from build123d import *
from OCP.BRepFilletAPI import BRepFilletAPI_MakeChamfer

# Parameters (mm, degrees)
SKETCH_1_W          = 46
SKETCH_1_H          = 21.3
EXTRUDE_1_DEPTH     = 2
SKETCH_2_R          = 8.3
CUT_EXTRUDE_1_DEPTH = 26.424840216
SKETCH_3_W          = 8
SKETCH_3_H          = 3
CUT_EXTRUDE_2_DEPTH = 26.424840216
SKETCH_4_W          = 5
SKETCH_4_H          = 4
CUT_EXTRUDE_3_DEPTH = 26.424840216
SKETCH_5_W          = 3
SKETCH_5_H          = 2
SKETCH_5_W_2        = 2
SKETCH_5_H_2        = 3
CUT_EXTRUDE_4_DEPTH = 1
SKETCH_8_W          = 46
SKETCH_8_H          = 2
EXTRUDE_2_DEPTH     = 5
SKETCH_9_W          = 46
SKETCH_9_H          = 14
EXTRUDE_3_DEPTH     = 3
HOLE_WIZARD_M3_1_D  = 3.4
HOLE_WIZARD_M4_1_D  = 4.5
RIB_1_REACH         = 34.754
SKETCH_13_WALL_W    = 79.877255328
SKETCH_13_WALL_H    = 8
CHAMFER_1_SIZE      = 8
CHAMFER_1_SIZE2     = 4.618802154


with BuildPart() as part:
    # 草圖1 → 填料-伸長1 (new body)
    with BuildSketch(Plane.XY):
        Rectangle(SKETCH_1_W, SKETCH_1_H)
    extrude(amount=EXTRUDE_1_DEPTH)

    # 草圖2 → 除料-伸長1 (cut, through all)
    with BuildSketch(Plane.XY.offset(2)):
        with Locations((-12.7, 0)):
            Circle(SKETCH_2_R)
        with Locations((12.7, 0)):
            Circle(SKETCH_2_R)
    extrude(amount=-CUT_EXTRUDE_1_DEPTH, mode=Mode.SUBTRACT)

    # 草圖3 → 除料-伸長2 (cut, through all)
    with BuildSketch(Plane.XY.offset(2)):
        with Locations((0, 9.15)):
            Rectangle(SKETCH_3_W, SKETCH_3_H)
    extrude(amount=-CUT_EXTRUDE_2_DEPTH, mode=Mode.SUBTRACT)

    # 草圖4 → 除料-伸長3 (cut, through all)
    with BuildSketch(Plane.XY.offset(2)):
        with Locations((0, -5.5)):
            Rectangle(SKETCH_4_W, SKETCH_4_H)
    extrude(amount=-CUT_EXTRUDE_3_DEPTH, mode=Mode.SUBTRACT)

    # 草圖5 → 除料-伸長4 (cut)
    with BuildSketch(Plane.XY.offset(2)):
        with Locations((4, -6.5)):
            Rectangle(SKETCH_5_W, SKETCH_5_H)
        with Locations((-5.5, 8.65)):
            Rectangle(SKETCH_5_W_2, SKETCH_5_H_2)
        with Locations((5.5, 8.65)):
            Rectangle(SKETCH_5_W_2, SKETCH_5_H_2)
    extrude(amount=-CUT_EXTRUDE_4_DEPTH, mode=Mode.SUBTRACT)

    # 草圖8 → 填料-伸長2 (add)
    with BuildSketch(Plane.XZ.offset(10.65)):
        with Locations((0, 1)):
            Rectangle(SKETCH_8_W, SKETCH_8_H)
    extrude(amount=EXTRUDE_2_DEPTH)

    # 草圖9 → 填料-伸長3 (add)
    with BuildSketch(Plane.XZ.offset(15.65)):
        with Locations((0, 7)):
            Rectangle(SKETCH_9_W, SKETCH_9_H)
    extrude(amount=EXTRUDE_3_DEPTH)

    # M3 餘隙孔1 (through all)
    with Locations(Plane.XY.offset(2)):
        with Locations((20.7, 8.6), (-20.7, -8.6), (-20.7, 8.6), (20.7, -8.6)):
            Hole(HOLE_WIZARD_M3_1_D / 2)

    # M4 餘隙孔1 (through all)
    with Locations(Plane(origin=(0, -15.65, 0), x_dir=(1, 0, 0), z_dir=(0, 1, 0))):
        with Locations((12, -10), (-12, -10)):
            Hole(HOLE_WIZARD_M4_1_D / 2)

    # 草圖13 wall → 肋材1 (add, up to next)
    with BuildSketch(Plane(origin=(0, -14.15, 8), x_dir=(0, -0.242535625036, 0.970142500145), z_dir=(0, -0.970142500145, -0.242535625036)), mode=Mode.PRIVATE) as rib_1_sk1:
        Rectangle(SKETCH_13_WALL_W, SKETCH_13_WALL_H)
    rib_1_tool1 = extrude(rib_1_sk1.sketch, amount=RIB_1_REACH, mode=Mode.PRIVATE) - part.part
    add(rib_1_tool1.solids().sort_by_distance((0, -14.15, 8))[0])

    # 導角1: one chamfer whose edges measure the first distance from different faces: ONE call of the kernel's chamfer builder (chamfer() names one face for all edges)
    chamfer_1_edges_1 = [part.edges().sort_by_distance(p)[0] for p in [
        (-23, -17.15, 14),
    ]]
    chamfer_1_side_1 = [part.faces().sort_by_distance(p)[0] for p in [
        (-23, 10.325270882, 1),
    ]]
    chamfer_1_edges_2 = [part.edges().sort_by_distance(p)[0] for p in [
        (23, -17.15, 14),
    ]]
    chamfer_1_side_2 = [part.faces().sort_by_distance(p)[0] for p in [
        (23, 10.325270882, 1),
    ]]
    chamfer_1 = BRepFilletAPI_MakeChamfer(part.part.solid().wrapped)
    for e in chamfer_1_edges_1:
        chamfer_1.Add(CHAMFER_1_SIZE, CHAMFER_1_SIZE2, e.wrapped, chamfer_1_side_1[0].wrapped)  # the first distance lies on this face
    for e in chamfer_1_edges_2:
        chamfer_1.Add(CHAMFER_1_SIZE, CHAMFER_1_SIZE2, e.wrapped, chamfer_1_side_2[0].wrapped)  # the first distance lies on this face
    add(Compound.cast(chamfer_1.Shape()), mode=Mode.REPLACE)


solid = part.part
Verification items for the finished model (mm, model axes). A direction names the side the tool comes from. Round coordinates to 2 decimals unless told otherwise and drop trailing zeros. Loops run counter-clockwise (first coordinate to the right, second up) from the corner with the lowest first, then second, coordinate; pieces in that order, holes last. Notation, with made-up numbers: M -26.5,62 L 10.5,62 A17 cw 10.5,81 Z; hole C 55.25,4 d4. An arc over 180 degrees is marked long. Write each question's results on one line, items separated by ' | '.
1) Section check D-D on x = 12. Record the boundary of the cut face in (y, z), then the cut area to 3 significant figures.
Checks:
outline: M -18.65,0 L -8.27,0 L -8.27,2 L -15.65,2 L -15.65,7.75 L -18.65,7.75 Z; M -18.65,12.25 L -15.65,12.25 L -15.65,14 L -18.65,14 Z; M 8.27,0 L 10.65,0 L 10.65,2 L 8.27,2 Z | area: 48.0 mm2
2) Gauge pin test, flat ends, axial feed: P1, Ø7, axis at x = -12, z = 10, coming from the +Y side; P2, Ø3, axis at x = -2.5, y = -9, coming from the +Z side; P3, Ø2, axis at x = 1.5, z = 1.5, coming from the +Y side. Record the tip position at first contact, or that the pin passes through.
Checks:
P1: stops at y = -15.65 | P2: stops at z = 2 | P3: stops at y = 7.65
3) Section check B-B on z = 9. Record the boundary of the cut face in (x, y).
Checks:
outline: M -21.27,-18.65 L -14.02,-18.65 L -14.02,-15.65 L -21.27,-15.65 Z; M -9.98,-18.65 L 9.98,-18.65 L 9.98,-15.65 L 4,-15.65 L 4,-14.4 L -4,-14.4 L -4,-15.65 L -9.98,-15.65 Z; M 14.02,-18.65 L 21.27,-18.65 L 21.27,-15.65 L 14.02,-15.65 Z
4) Access from +Z, -Z, +X, -X, +Y, -Y to the whole of each face (thin tool, end or side, straight path). Record for faces 4 (the flat face through (4, -15, 6)), 5 (the flat face through (4, 9, 1)), 6 (the flat face through (13, 10.65, 1)), 7 (the flat face through (5.5, 7.15, 1.5)), 8 (the flat face through (2.5, -5, 1)).
Checks:
face 4: +Z, +X, +Y | face 5: +Z, -Z, +Y | face 6: +Z, -Z, +X, -X, +Y | face 7: +Z | face 8: +Z, -Z
5) Section check C-C on y = -1.5. Record the boundary of the cut face in (x, z), then the cut area to 3 significant figures.
Checks:
outline: M -23,0 L -20.86,0 L -20.86,2 L -23,2 Z; M -4.54,0 L 4.54,0 L 4.54,2 L -4.54,2 Z; M 20.86,0 L 23,0 L 23,2 L 20.86,2 Z | area: 26.7 mm2
6) Scan lines: L1, parallel to X at y = -16.8, z = 10; L2, parallel to Y at x = 2, z = 0.5; L3, parallel to Z at x = -7, y = -9.5. Record each from-to range of solid material in increasing order. Write a range as from..to.
Checks:
L1: x = -20.69..-14.25, -9.75..9.75, 14.25..20.69 | L2: y = -18.65..-7.5, -3.5..7.65 | L3: z = 0..2
7) Mould release check, pull along Y, two halves, no side actions. Record for faces 1 (the flat face through (5.5, 10.15, 1.5)), 2 (the flat face through (0, -2, 2)), 3 (the flat face through (-14, -15.65, 8)): released by +Y, released by -Y, zero draft, split by the parting line, or undercut.
Checks:
face 1: undercut | face 2: zero draft | face 3: released by +Y
8) Section check A-A on x = -15.5. Record the boundary of the cut face in (y, z).
Checks:
outline: M -18.65,0 L -7.81,0 L -7.81,2 L -15.65,2 L -15.65,14 L -18.65,14 Z; M 7.81,0 L 10.65,0 L 10.65,2 L 7.81,2 Z
